Could you check a few things on this model? Use its own coordinates, in mm. Face numbers are marked on the shaded views. A direction names the side the tool comes from. Coordinates: 2 decimals unless noted, no trailing zeros. Loops run counter-clockwise (first coordinate to the right, second up) from the corner with the lowest first, then second, coordinate; pieces in that order, holes last. Notation, with made-up numbers: (53, -22.75) -> (78, -22.75) arc R20 ccw to (78, -5.75) -> close; hole circle Ø7 at (-11.75, 52). An arc over 180 degrees is marked (long way). One line per question, with ' | ' between items. Start each with the question number.
(1) Suppose I cut it at B-B (y = -205.5). Please give me the cut outline in (x, z), plus the area to 3 significant figures.
(2) If I drill on line 1 along Y through (x, z) = (-493, -22); line 2 along X through (y, z) = (314, -458); line 3 along X through (y, z) = (-166.5, -50.5), over which ranges is the centre line in solid material (lowest first)?
(3) If we mould it in two halves opening along Y, with no side actions, what happens to the marked faces 1, 2, 3 and 4? For each: pulls with the +Y half, pulls with the -Y half, needs draft (parallel to the pull), parting line crosses it, or undercut.
(4) Suppose I cut it at A-A (z = -83.5). Please give me the cut outline in (x, y).
(5) I'm going to push flat-ended pins straight in: pin 1 Ø8 at (x, y) = (404, -273) entering from -Z; pin 2 Ø15 at (x, y) = (216, -332) entering from -Z. Where does each tip first touch, or does it pass through?
(6) Suppose I cut it at D-D (x = -214). Please give me the cut outline in (y, z), plus the area to 3 significant figures.
(7) Which directions (+Z, -Z, +X, -X, +Y, -Y) give clear straight access to the entire face, cutting with the end or side of a thin tool? Please do the marked faces 5, 6, 7 and 8.
(8) Suppose I cut it at C-C (z = -618.5). Please give me the cut outline in (x, y), plus the area to 3 significant figures.
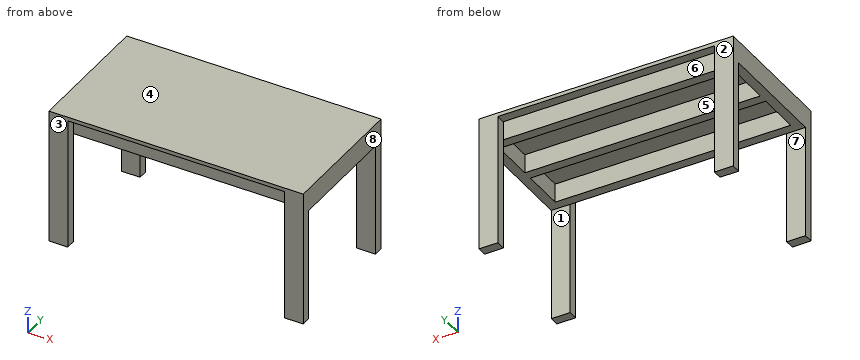
```python
from build123d import *

# Parameters (mm, degrees)
F0_W     = 1350
F0_H     = 710
F1_DEPTH = 20
F2_W     = 100
F2_H     = 50
F3_DEPTH = 700
F4_W     = 1250
F4_H     = 50
F5_DEPTH = 100


with BuildPart() as f1:
    # F0 (on Top) → F1 (new body)
    with BuildSketch(Plane.XY):
        Rectangle(F0_W, F0_H)
    extrude(amount=F1_DEPTH)

    # F2 (on face) → F3 (join)
    with BuildSketch(Plane(origin=(0, 0, 0), x_dir=(1, 0, 0), z_dir=(0, 0, -1))):
        with Locations((625, -330)):
            Rectangle(F2_W, F2_H)
        with Locations((-625, 330)):
            Rectangle(F2_W, F2_H)
        with Locations((625, 330)):
            Rectangle(F2_W, F2_H)
        with Locations((-625, -330)):
            Rectangle(F2_W, F2_H)
    extrude(amount=F3_DEPTH)

    # F4 (on face) → F5 (join)
    with BuildSketch(Plane(origin=(0, 0, 0), x_dir=(1, 0, 0), z_dir=(0, 0, -1))):
        Polygon((-625, 305), (-675, 305), (-675, -305), (-625, -305), (-625, -253.84596), (-625, -22.106195), (-625, 27.893805), (-625, 255), align=None)
        Polygon((-575, 305), (-625, 305), (-625, 255), (625, 255), (625, 305), (575, 305), align=None)
        Polygon((-625, -253.84596), (-625, -305), (-575, -305), (575, -305), (625, -305), (625, -253.84596), align=None)
        Polygon((625, 305), (625, 255), (625, 27.893805), (625, -22.106195), (625, -253.84596), (625, -305), (675, -305), (675, 305), align=None)
        with Locations((0, 2.893805)):
            Rectangle(F4_W, F4_H)
    extrude(amount=F5_DEPTH)


solid = f1.part
```
Checks:
1) outline: (-675, -100) -> (-625, -100) -> (-625, 0) -> (625, 0) -> (625, -100) -> (675, -100) -> (675, 20) -> (-675, 20) -> close | area: 37,000 mm^2
2) line 1: y = -305 to -255, -27.89 to 22.11, 253.85 to 305 | line 2: x = -675 to -575, 575 to 675 | line 3: x = -675 to -625, 625 to 675
3) face 1: undercut | face 2: pulls with the +Y half | face 3: pulls with the -Y half | face 4: needs draft
4) outline: (-675, -355) -> (-575, -355) -> (-575, -305) -> (575, -305) -> (575, -355) -> (675, -355) -> (675, 355) -> (575, 355) -> (575, 305) -> (-575, 305) -> (-575, 355) -> (-675, 355) -> close; hole (-625, -255) -> (625, -255) -> (625, -27.89) -> (-625, -27.89) -> close; hole (-625, 22.11) -> (625, 22.11) -> (625, 253.85) -> (-625, 253.85) -> close
5) pin 1: stops at z = -100 | pin 2: stops at z = 0
6) outline: (-355, 0) -> (-305, 0) -> (-305, -100) -> (-255, -100) -> (-255, 0) -> (-27.89, 0) -> (-27.89, -100) -> (22.11, -100) -> (22.11, 0) -> (253.85, 0) -> (253.85, -100) -> (305, -100) -> (305, 0) -> (355, 0) -> (355, 20) -> (-355, 20) -> close | area: 29,300 mm^2
7) face 5: -Z | face 6: -Z, +Y | face 7: -Z, +X, -X | face 8: +Z, -Z, +X, +Y, -Y
8) outline: (-675, -355) -> (-575, -355) -> (-575, -305) -> (-675, -305) -> close; (-675, 305) -> (-575, 305) -> (-575, 355) -> (-675, 355) -> close; (575, -355) -> (675, -355) -> (675, -305) -> (575, -305) -> close; (575, 305) -> (675, 305) -> (675, 355) -> (575, 355) -> close | area: 20,000 mm^2
